from build123d import *

# Parameters (mm, degrees)
CHAMFER1_SIZE = 1


with BuildPart() as part:
    # Sketch1 → Revolve3 (revolve)
    with BuildSketch(Plane(origin=(0, 0, 0), x_dir=(0, 0, -1), z_dir=(1, 0, 0))):
        with BuildLine():
            Line((-458.414283312, 54), (-458.414283312, 63.3349))
            Line((-458.414283312, 63.3349), (-442.555821638, 63.3349))
            Line((-442.555821638, 63.3349), (-442.555821638, 54))
            ThreePointArc((-442.555821638, 54), (-443.54515622, 27.008055426), (-443.875, 0))
            Line((-443.875, 0), (-451.375, 0))
            ThreePointArc((-451.375, 0), (-453.142234121, 27.228438761), (-458.414283312, 54))
        make_face()
    revolve(axis=Axis((0, 0, 662.018), (0, 0, -1)))

    # Chamfer1
    chamfer1_edges = [part.edges().sort_by_distance(p)[0] for p in [
        (0, -63.3349, 442.555821638),
        (0, -63.3349, 458.414283312),
    ]]
    chamfer(chamfer1_edges, length=CHAMFER1_SIZE)


solid = part.part
Build history of the part. All positions in model axes, mm. Coordinates: 2 decimals unless noted, no trailing zeros. Order: outer loops, then holes, each group sorted by start corner. A loop starts at its lowest first (then second) coordinate and runs counter-clockwise, first axis right, second up. Notation, with made-up numbers: (25.25, -37.5) - (46.25, -37.5) arc R22 ccw to (46.25, -10.5) - close; hole circle Ø10 at (-10, 50). An arc over 180 degrees is marked (long way). Write item = value, one per line. Start each with the question number.
1) Saw through at C-C on z = 448.5. Write the cut outline in (x, y).
2) Wall check: line 1 along X through (y, z) = (11, 444.75); line 2 along X through (y, z) = (-0.5, 446.5); line 3 along Z through (x, y) = (49, 16.5). Give the ranges that are in metal, low to high. Write a range as from..to.
3) Saw through at B-B on x = 0. Write the cut outline in (y, z) (3 decimals), then the cut area to 3 significant figures.
4) Flat gauge pins, fed straight in: pin 1 Ø6 at (y, z) = (43, 449) entering from -X; pin 2 Ø1 at (x, z) = (-37, 454.5) entering from +Y; pin 3 Ø6 at (y, z) = (28, 445) entering from -X. Where does each tip first touch, or does it go through?
5) Saw through at A-A on y = 0. Write the cut outline in (x, z), then the cut area to 3 significant figures.
From the geometry:
q1.outline = circle Ø126.67 at (0, 0)
q2.line_1 = -62.37..62.37
q2.line_2 = -63.33..63.33
q2.line_3 = 442.67..457.82
q3.outline = (-63.335, 443.556) - (-62.335, 442.556) - (-54, 442.556) arc R1105.893 cw to (54, 442.556) - (62.335, 442.556) - (63.335, 443.556) - (63.335, 457.414) - (62.335, 458.414) - (54, 458.414) arc R210.643 cw to (-54, 458.414) - (-62.335, 458.414) - (-63.335, 457.414) - close
q3.area = 1,400 mm^2
q4.pin_1 = -49.11
q4.pin_2 = 51.76
q4.pin_3 = -58.19
q5.outline = (-63.33, 443.56) - (-62.33, 442.56) - (-54, 442.56) arc R1105.89 cw to (54, 442.56) - (62.33, 442.56) - (63.33, 443.56) - (63.33, 457.41) - (62.33, 458.41) - (54, 458.41) arc R210.64 cw to (-54, 458.41) - (-62.33, 458.41) - (-63.33, 457.41) - close
q5.area = 1,400 mm^2
